Here's the drawing with two shaded views (mm, measured from the low corner). I have some questions. A direction names the side the tool comes from. Round coordinates to 2 decimals unless told otherwise and drop trailing zeros. Order: outer loops, then holes, each group sorted by start corner. A loop starts at its lowest first (then second) coordinate and runs counter-clockwise, first axis right, second up. Notation, with made-up numbers: (10, 86.25) -> (49, 86.25) arc R18 ccw to (49, 120.25) -> close; hole circle Ø7 at (37.5, -36.75). An arc over 180 degrees is marked (long way). Answer in a Markdown table with one row per item.
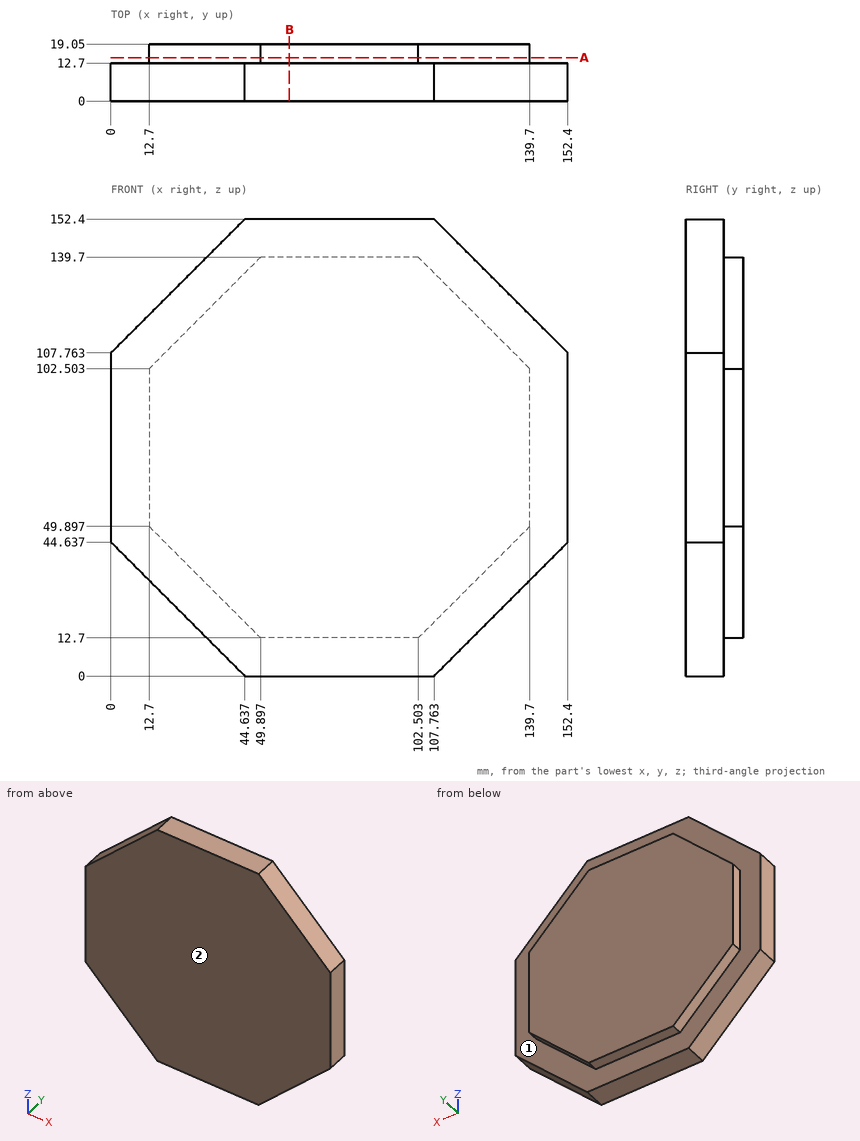
1. For pin 1 Ø2 at (x, y) = (15.5, 16) entering from -Z; pin 2 Ø1.5 at (y, z) = (14, 53.5) entering from -X; pin 3 Ø6 at (y, z) = (9, 115.5) entering from +X, each with a flat end and sliding along its axis, tell me the tip position at first contact or that it passes through.
Numbers:
| item | result |
|---|---|
| pin 1 | stops at z = 46.1 |
| pin 2 | stops at x = 12.7 |
| pin 3 | stops at x = 147.66 |
2. For the marked faces 1 and 2, which set-ups out of +Z, -Z, +X, -X, +Y, -Y let a thin tool reach every point of the face, with its end or its side?
Numbers:
| item | result |
|---|---|
| face 1 | +Y |
| face 2 | +Z, -Z, +X, -X, -Y |
3. Suppose I cut it at B-B on x = 59.5. Write out the boundary of the cut face in (y, z), then the cut area to 3 significant figures.
Numbers:
| item | result |
|---|---|
| outline | (0, 0) -> (12.7, 0) -> (12.7, 12.7) -> (19.05, 12.7) -> (19.05, 139.7) -> (12.7, 139.7) -> (12.7, 152.4) -> (0, 152.4) -> close |
| area | 2,740 mm2 |
4. Suppose I cut it at A-A on y = 14.5. Write out the boundary of the cut face in (x, z), then the cut area to 3 significant figures.
Numbers:
| item | result |
|---|---|
| outline | (12.7, 49.9) -> (49.9, 12.7) -> (102.5, 12.7) -> (139.7, 49.9) -> (139.7, 102.5) -> (102.5, 139.7) -> (49.9, 139.7) -> (12.7, 102.5) -> close |
| area | 13,400 mm2 |
5. Please list where these lines run through material, in increasing order: line 1 along Y through (x, z) = (8, 69); line 2 along Z through (x, y) = (98, 15.75); line 3 along X through (y, z) = (2, 26.5) (1 decimal).
Numbers:
| item | result |
|---|---|
| line 1 | y = 0 to 12.7 |
| line 2 | z = 12.7 to 139.7 |
| line 3 | x = 18.1 to 134.3 |
